Design review of the part built by this model. Coordinates are the model's own, in mm. A direction names the side the tool comes from. Coordinates: 2 decimals unless noted, no trailing zeros. Loops run counter-clockwise (first coordinate to the right, second up) from the corner with the lowest first, then second, coordinate; pieces in that order, holes last. Notation, with made-up numbers: (42, -8) - (85, -8) arc R33 ccw to (85, 31) - close; hole circle Ø2 at (89.25, 40). An arc over 180 degrees is marked (long way). Answer in a Markdown table with one row per item. Add a question column.
(1) The part is to be moulded in two halves that separate along X. For faces 1 (the face through (3.07, 1.05, 2.42)), 2 (the face through (-3.07, 1.05, 2.42)), 3 (the face through (0, -1.25, 2)), say which applies: released by +X, released by -X, zero draft, split by the parting line, or undercut.
(2) Clearance check with a flat-ended pin moving along its axis: pin 1 (0.8 mm diameter, centred on x = 0, y = 0, fed in from -Z). State where the tip first meets the part, or that it passes through.
(3) We need section C-C, the plane x = -0.25. Write out the cut boundary in (y, z).
(4) To check wall thickness, follow L1, parallel to X at y = 0.35, z = 0.6; L2, parallel to Y at x = -1, z = 1.65; L3, parallel to Z at x = 3, y = 1.3. State the ranges of each line that lie inside material, in increasing order. Write a range as [from, to].
(5) For faces 4 (the face through (-3.07, -1.05, 2.42)), 5 (the face through (3.07, -1.05, 2.42)), 6 (the face through (4, 0, 0.8)), 7 (the face through (0, 1.25, 2)), 8 (the face through (0, -1.5, 2)), list the 3-axis set-ups (+Z, -Z, +X, -X, +Y, -Y) from which the entire face can be reached by the end or side of a thin tool; tool diameter is ignored.
(6) We need section D-D, the plane y = 0.15. Write out the cut boundary in (x, z), plus the area to 3 significant figures.
(7) We need section A-A, the plane z = 0.6. Write out the cut boundary in (x, y), plus the area to 4 significant figures.
from build123d import *

# Parameters (mm, degrees)
F0_W     = 7
F0_H     = 3
F0_W_2   = 2.5
F0_H_2   = 2.5
F1_DEPTH = 4
F0_W_3   = 1.5
F2_DEPTH = 0.8
F3_R     = 1.49999
F4_DEPTH = 3.6


# Not quite as in the source:
# - a fillet or chamfer is up to 0.001 mm smaller than in the source, because OpenCascade refuses the exact size


with BuildPart() as f1:
    # F0 (on Top) → F1 (new body)
    with BuildSketch(Plane.XY):
        Rectangle(F0_W, F0_H)
        Rectangle(F0_W_2, F0_H_2, mode=Mode.SUBTRACT)
        Rectangle(F0_W_2, F0_H_2)
    extrude(amount=F1_DEPTH)

    # F0 (on Top) → F2 (join)
    with BuildSketch(Plane.XY):
        with Locations((-4.25, 0)):
            Rectangle(F0_W_3, F0_H)
        with Locations((4.25, 0)):
            Rectangle(F0_W_3, F0_H)
    extrude(amount=F2_DEPTH)

    # F3 (radius 1.5 in the source; OpenCascade refuses exactly that, so slightly less here)
    f3_edges = [f1.edges().sort_by_distance(p)[0] for p in [
        (-3.5, 1.5, 2.4),
        (-3.5, -1.5, 2.4),
        (3.5, -1.5, 2.4),
        (3.5, 1.5, 2.4),
    ]]
    fillet(f3_edges, radius=F3_R)

    # F0 (on Top) → F4 (cut)
    with BuildSketch(Plane.XY):
        Rectangle(F0_W_2, F0_H_2)
    extrude(amount=F4_DEPTH, mode=Mode.SUBTRACT)


solid = f1.part
Responses:
| question | item | result |
|---|---|---|
| 1 | face 1 | released by +X |
| 1 | face 2 | released by -X |
| 1 | face 3 | undercut |
| 2 | pin 1 | stops at z = 3.6 |
| 3 | outline | (-1.5, 0) - (-1.25, 0) - (-1.25, 3.6) - (1.25, 3.6) - (1.25, 0) - (1.5, 0) - (1.5, 4) - (-1.5, 4) - close |
| 4 | L1 | x = [-5, -1.25], [1.25, 5] |
| 4 | L2 | y = [-1.5, -1.25], [1.25, 1.5] |
| 4 | L3 | z = [0, 0.8] |
| 5 | face 4 | +Z, -X, -Y |
| 5 | face 5 | +Z, +X, -Y |
| 5 | face 6 | +Z, +X, -Y |
| 5 | face 7 | -Z |
| 5 | face 8 | +Z, -Z, +X, -X, -Y |
| 6 | outline | (-5, 0) - (-1.25, 0) - (-1.25, 3.6) - (1.25, 3.6) - (1.25, 0) - (5, 0) - (5, 0.8) - (3.49, 0.8) - (3.49, 4) - (-3.49, 4) - (-3.49, 0.8) - (-5, 0.8) - close |
| 6 | area | 21.4 mm2 |
| 7 | outline | (-5, -1.5) - (5, -1.5) - (5, 1.5) - (-5, 1.5) - close; hole (-1.25, -1.25) - (1.25, -1.25) - (1.25, 1.25) - (-1.25, 1.25) - close |
| 7 | area | 23.75 mm2 |
